```python
from build123d import *

# Parameters (mm, degrees)
CYLINDER020_R     = 2
CYLINDER020_DEPTH = 100
BOX011_W          = 20
BOX011_H          = 7.2
BOX011_DEPTH      = 10
CYLINDER016_R     = 0.8
CYLINDER016_DEPTH = 20
CYLINDER017_R     = 0.8
CYLINDER017_DEPTH = 20
CYLINDER018_R     = 0.8
CYLINDER018_DEPTH = 20
CYLINDER019_R     = 0.8
CYLINDER019_DEPTH = 20
BOX010_W          = 39.8
BOX010_H          = 1
BOX010_DEPTH      = 0.8
BOX009_W          = 39.8
BOX009_H          = 1
BOX009_DEPTH      = 0.8
BOX007_W          = 20
BOX007_H          = 7.2
BOX007_DEPTH      = 10
BOX006_W          = 42
BOX006_H          = 44
BOX006_DEPTH      = 1
BOX005_W          = 39.8
BOX005_H          = 41.8
BOX005_DEPTH      = 1


with BuildPart() as zylinder020:
    # Cylinder020 → Cylinder020 (new body)
    with BuildSketch(Plane(origin=(30, 21, -50), x_dir=(1, 0, 0), z_dir=(0, 0, 1))):
        Circle(CYLINDER020_R)
    extrude(amount=CYLINDER020_DEPTH)


with BuildPart() as obj1:
    # Box011 → Box011 (new body)
    with BuildSketch(Plane(origin=(-12.4, 22.4, 0), x_dir=(1, 0, 0), z_dir=(0, 0, 1))):
        with Locations((10, 3.6)):
            Rectangle(BOX011_W, BOX011_H)
    extrude(amount=BOX011_DEPTH)


with BuildPart() as zylinder016:
    # Cylinder016 → Cylinder016 (new body)
    with BuildSketch(Plane(origin=(37.5, 2.5, -10), x_dir=(1, 0, 0), z_dir=(0, 0, 1))):
        Circle(CYLINDER016_R)
    extrude(amount=CYLINDER016_DEPTH)


with BuildPart() as zylinder017:
    # Cylinder017 → Cylinder017 (new body)
    with BuildSketch(Plane(origin=(2.5, 2.5, -10), x_dir=(1, 0, 0), z_dir=(0, 0, 1))):
        Circle(CYLINDER017_R)
    extrude(amount=CYLINDER017_DEPTH)


with BuildPart() as zylinder018:
    # Cylinder018 → Cylinder018 (new body)
    with BuildSketch(Plane(origin=(37.5, 39.5, -10), x_dir=(1, 0, 0), z_dir=(0, 0, 1))):
        Circle(CYLINDER018_R)
    extrude(amount=CYLINDER018_DEPTH)


with BuildPart() as compound006:
    # Cylinder019 → Cylinder019 (new body)
    with BuildSketch(Plane(origin=(2.5, 39.5, -10), x_dir=(1, 0, 0), z_dir=(0, 0, 1))):
        Circle(CYLINDER019_R)
    extrude(amount=CYLINDER019_DEPTH)

    # Compound006: union Zylinder016, Zylinder017, Zylinder018
    add(zylinder016.part)
    add(zylinder017.part)
    add(zylinder018.part)


with BuildPart() as obj2:
    # Box010 → Box010 (new body)
    with BuildSketch(Plane(origin=(0.1, 0.1, 0.7), x_dir=(1, 0, 0), z_dir=(0, 0, 1))):
        with Locations((19.9, 0.5)):
            Rectangle(BOX010_W, BOX010_H)
    extrude(amount=BOX010_DEPTH)


with BuildPart() as compound003:
    # Box009 → Box009 (new body)
    with BuildSketch(Plane(origin=(0.1, 40.9, 0.7), x_dir=(1, 0, 0), z_dir=(0, 0, 1))):
        with Locations((19.9, 0.5)):
            Rectangle(BOX009_W, BOX009_H)
    extrude(amount=BOX009_DEPTH)

    # Compound003: union obj2
    add(obj2.part)


with BuildPart() as obj3:
    # Box007 → Box007 (new body)
    with BuildSketch(Plane(origin=(-12.4, 12.4, 0), x_dir=(1, 0, 0), z_dir=(0, 0, 1))):
        with Locations((10, 3.6)):
            Rectangle(BOX007_W, BOX007_H)
    extrude(amount=BOX007_DEPTH)


with BuildPart() as obj4:
    # Box006 → Box006 (new body)
    with BuildSketch(Plane(origin=(-1, -1, 2.5), x_dir=(1, 0, 0), z_dir=(0, 0, 1))):
        with Locations((21, 22)):
            Rectangle(BOX006_W, BOX006_H)
    extrude(amount=BOX006_DEPTH)


with BuildPart() as lowerparthole:
    # Box005 → Box005 (new body)
    with BuildSketch(Plane(origin=(0.1, 0.1, 1.5), x_dir=(1, 0, 0), z_dir=(0, 0, 1))):
        with Locations((19.9, 20.9)):
            Rectangle(BOX005_W, BOX005_H)
    extrude(amount=BOX005_DEPTH)

    # Fusion001: union obj4
    add(obj4.part)

    # Cut003: cut obj3
    add(obj3.part, mode=Mode.SUBTRACT)

    # Fusion003: union Compound003
    add(compound003.part)

    # Cut008: cut Compound006
    add(compound006.part, mode=Mode.SUBTRACT)

    # Cut009: cut obj1
    add(obj1.part, mode=Mode.SUBTRACT)

    # Cut010: cut Zylinder020
    add(zylinder020.part, mode=Mode.SUBTRACT)


solid = lowerparthole.part
```
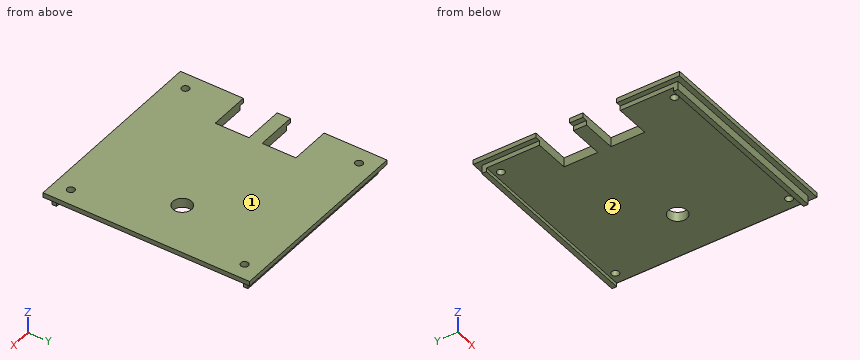
Can you work these out from the model? Positions are in its coordinate system, mm. Face numbers are marked on the shaded views. Coordinates: 2 decimals unless noted, no trailing zeros. Loops run counter-clockwise (first coordinate to the right, second up) from the corner with the lowest first, then second, coordinate; pieces in that order, holes last. Notation, with made-up numbers: (88, 52.25) -> (139, 52.25) arc R30 cw to (139, 80.25) -> close; hole circle Ø5 at (-17, -15). An arc over 180 degrees is marked (long way). Answer as a JSON object with one key per item and string values.
1) Imagine slicing it at B-B (y = 21). Please give me the cut outline in (x, z).
Results:
{"outline": "(-1, 2.5) -> (0.1, 2.5) -> (0.1, 1.5) -> (28, 1.5) -> (28, 3.5) -> (-1, 3.5) -> close; (32, 1.5) -> (39.9, 1.5) -> (39.9, 2.5) -> (41, 2.5) -> (41, 3.5) -> (32, 3.5) -> close"}
2) For P1, Ø0.6, axis at x = 28, z = 1, coming from the -Y side; P2, Ø1, axis at x = 2.5, y = 39.5, coming from the +Z side; P3, Ø8, axis at x = 20, y = 12, coming from the -Z side; P4, Ø1.4, axis at y = 19, z = 1.5, coming from the +X side, each with a flat end and sliding along its axis, tell me the tip position at first contact or that it passes through.
Results:
{"P1": "stops at y = 0.1", "P2": "passes through", "P3": "stops at z = 1.5", "P4": "stops at x = 39.9"}
3) Imagine slicing it at C-C (y = 39.5). Please give me the cut outline in (x, z).
Results:
{"outline": "(-1, 2.5) -> (0.1, 2.5) -> (0.1, 1.5) -> (1.7, 1.5) -> (1.7, 3.5) -> (-1, 3.5) -> close; (3.3, 1.5) -> (36.7, 1.5) -> (36.7, 3.5) -> (3.3, 3.5) -> close; (38.3, 1.5) -> (39.9, 1.5) -> (39.9, 2.5) -> (41, 2.5) -> (41, 3.5) -> (38.3, 3.5) -> close"}
4) Thinking about a two-plate mould opening in Y: for the marked faces 1 and 2, which applies, pulls with the +Y half, pulls with the -Y half, needs draft (parallel to the pull), parting line crosses it, or undercut?
Results:
{"face 1": "needs draft", "face 2": "undercut"}
5) Imagine slicing it at A-A (x = 37.5). Please give me the cut outline in (y, z), then the cut area to 3 significant figures.
Results:
{"outline": "(-1, 2.5) -> (0.1, 2.5) -> (0.1, 0.7) -> (1.1, 0.7) -> (1.1, 1.5) -> (1.7, 1.5) -> (1.7, 3.5) -> (-1, 3.5) -> close; (3.3, 1.5) -> (38.7, 1.5) -> (38.7, 3.5) -> (3.3, 3.5) -> close; (40.3, 1.5) -> (40.9, 1.5) -> (40.9, 0.7) -> (41.9, 0.7) -> (41.9, 2.5) -> (43, 2.5) -> (43, 3.5) -> (40.3, 3.5) -> close", "area": "81.0 mm^2"}
6) Imagine slicing it at D-D (x = 11). Please give me the cut outline in (y, z), then the cut area to 3 significant figures.
Results:
{"outline": "(-1, 2.5) -> (0.1, 2.5) -> (0.1, 0.7) -> (1.1, 0.7) -> (1.1, 1.5) -> (40.9, 1.5) -> (40.9, 0.7) -> (41.9, 0.7) -> (41.9, 2.5) -> (43, 2.5) -> (43, 3.5) -> (-1, 3.5) -> close", "area": "87.4 mm^2"}
7) If I drill on line 1 (Y direction, x = 37.5, z = 2.7); line 2 (Y direction, x = 37.5, z = 2); line 3 (X direction, y = 2.5, z = 2.4), over which ranges is the centre line in solid material (lowest first)?
Results:
{"line 1": "y = -1 to 1.7, 3.3 to 38.7, 40.3 to 43", "line 2": "y = 0.1 to 1.7, 3.3 to 38.7, 40.3 to 41.9", "line 3": "x = 0.1 to 1.7, 3.3 to 36.7, 38.3 to 39.9"}
